Geometry check sheet. Reference: the model listing, model coordinates, mm. A direction names the side the tool comes from. Give positions to 0.01 mm unless a question says otherwise; leave off trailing zeros. Write each loop counter-clockwise with the first axis right and the second up, starting at its lowest first coordinate (ties: lowest second). Pieces come first, ordered by that corner, then holes. Notation, with made-up numbers: (15, -25) -> (35, -25) arc R20 cw to (35, -18) -> close; hole circle Ø8 at (13.25, -33). An arc over 180 degrees is marked (long way). One line per item, written item: value.
from build123d import *

# Parameters (mm, degrees)
SKETCH_2_W          = 38
SKETCH_2_H          = 38
SKETCH_2_R          = 1.15
EXTRUDE_1_DEPTH     = 3.15
EXTRUDE_START       = 3.15
SKETCH_3_W          = 13
SKETCH_3_H          = 13
EXTRUDE_2_DEPTH     = 3.15
EXTRUDE_START_2     = 6.3
SKETCH_4_R          = 6.5
EXTRUDE_3_DEPTH     = 14
CUT_EXTRUDE_START   = 9
SKETCH_5_R          = 32.561017026
SKETCH_5_R_2        = 6
CUT_EXTRUDE_1_DEPTH = 5
SKETCH_6_W          = 10
SKETCH_6_H          = 4.7
EXTRUDE_4_DEPTH     = 6.2
CHAMFER_1_SIZE      = 0.5


with BuildPart() as part:
    # 草图2 → 凸台-拉伸1 (new body)
    with BuildSketch(Plane(origin=(0, 0, 0), x_dir=(1, 0, 0), z_dir=(0, 1, 0))):
        Rectangle(SKETCH_2_W, SKETCH_2_H)
        with Locations((14.25, 14.25)):
            Circle(SKETCH_2_R, mode=Mode.SUBTRACT)
        with Locations((-14.25, 14.25)):
            Circle(SKETCH_2_R, mode=Mode.SUBTRACT)
        with Locations((14.25, -14.25)):
            Circle(SKETCH_2_R, mode=Mode.SUBTRACT)
        with Locations((-14.25, -14.25)):
            Circle(SKETCH_2_R, mode=Mode.SUBTRACT)
    extrude(amount=EXTRUDE_1_DEPTH)

    # 草图3 → 凸台-拉伸2 (add)
    with BuildSketch(Plane(origin=(0, 0, 0), x_dir=(1, 0, 0), z_dir=(0, 1, 0)).offset(EXTRUDE_START)):
        with BuildLine():
            Line((-6.5, -2), (-6.5, 2))
            Line((-6.5, 2), (-9, 2))
            ThreePointArc((-9, 2), (-11, 0), (-9, -2))
            Line((-9, -2), (-6.5, -2))
        make_face()
        Rectangle(SKETCH_3_W, SKETCH_3_H)
        with BuildLine():
            ThreePointArc((9, -2), (11, 0), (9, 2))
            Line((9, 2), (6.5, 2))
            Line((6.5, 2), (6.5, -2))
            Line((6.5, -2), (9, -2))
        make_face()
    extrude(amount=EXTRUDE_2_DEPTH)

    # 草图4 → 凸台-拉伸3 (add)
    with BuildSketch(Plane(origin=(0, 0, 0), x_dir=(1, 0, 0), z_dir=(0, 1, 0)).offset(EXTRUDE_START_2)):
        Circle(SKETCH_4_R)
    extrude(amount=EXTRUDE_3_DEPTH)

    # 草图5 → 切除-拉伸1 (cut)
    with BuildSketch(Plane(origin=(0, 0, 0), x_dir=(1, 0, 0), z_dir=(0, 1, 0)).offset(CUT_EXTRUDE_START)):
        Circle(SKETCH_5_R)
        Circle(SKETCH_5_R_2, mode=Mode.SUBTRACT)
    extrude(amount=CUT_EXTRUDE_1_DEPTH, mode=Mode.SUBTRACT)

    # 草图6 → 凸台-拉伸4 (add)
    with BuildSketch(Plane(origin=(0, 0, 0), x_dir=(1, 0, 0), z_dir=(0, 1, 0))):
        with Locations((0, -12.35)):
            Rectangle(SKETCH_6_W, SKETCH_6_H)
    extrude(amount=-EXTRUDE_4_DEPTH)

    # 倒角1
    chamfer_1_edges = [part.edges().sort_by_distance(p)[0] for p in [
        (-6.5, 20.3, 0),
    ]]
    chamfer(chamfer_1_edges, length=CHAMFER_1_SIZE)


solid = part.part
1) Depth check by flat-ended pin: pin 1 Ø0.9 at (y, z) = (5, -4.5) entering from -X; pin 2 Ø3 at (x, y) = (-7.5, 5.5) entering from -Z; pin 3 Ø5 at (x, y) = (2, -4.5) entering from +Z. Enter the tip coordinate at first touch or a pass-through.
Verdict:
pin 1: x = -6.5
pin 2: z = -6.5
pin 3: z = 14.7
2) Sectioned sample at B-B on x = 14.25. Record the cut outline in (y, z).
Verdict:
outline: (0, -19) -> (3.15, -19) -> (3.15, -15.4) -> (0, -15.4) -> close; (0, -13.1) -> (3.15, -13.1) -> (3.15, 13.1) -> (0, 13.1) -> close; (0, 15.4) -> (3.15, 15.4) -> (3.15, 19) -> (0, 19) -> close
3) Sectioned sample at D-D on y = 11.5. Record the cut outline in (x, z), plus the area to 3 significant figures.
Verdict:
outline: circle Ø12 at (0, 0)
area: 113 mm^2
4) Mould release check, pull along Z, two halves, no side actions. Record for faces 6 (the flat face through (2, 9, 6)), 7 (the flat face through (-8, 5, 2)), 8 (the cylindrical face through (-15.4, 1.6, -14.3)): released by +Z, released by -Z, zero draft, split by the parting line, or undercut.
Verdict:
face 6: zero draft
face 7: released by +Z
face 8: undercut
5) Sectioned sample at C-C on z = 0. Record the cut outline in (x, y).
Verdict:
outline: (-19, 0) -> (19, 0) -> (19, 3.15) -> (11, 3.15) -> (11, 6.3) -> (6.5, 6.3) -> (6.5, 9) -> (6, 9) -> (6, 14) -> (6.5, 14) -> (6.5, 19.8) -> (6, 20.3) -> (-6, 20.3) -> (-6.5, 19.8) -> (-6.5, 14) -> (-6, 14) -> (-6, 9) -> (-6.5, 9) -> (-6.5, 6.3) -> (-11, 6.3) -> (-11, 3.15) -> (-19, 3.15) -> close
6) Sectioned sample at A-A on z = -14.25. Record the cut outline in (x, y), plus the area to 3 significant figures.
Verdict:
outline: (-19, 0) -> (-15.4, 0) -> (-15.4, 3.15) -> (-19, 3.15) -> close; (-13.1, 0) -> (13.1, 0) -> (13.1, 3.15) -> (-13.1, 3.15) -> close; (15.4, 0) -> (19, 0) -> (19, 3.15) -> (15.4, 3.15) -> close
area: 105 mm^2
7) Tool access check on faces 1 (the flat face through (-7, 6.3, -1)), 2 (the cylindrical face through (-5.158, 16.859, 3.955)), 3 (the flat face through (-5, -3, 12)), 4 (the flat face through (8, 5, -2)), 5 (the cylindrical face through (-6, 11, 0)). Record the directions out of +Z, -Z, +X, -X, +Y, -Y that give a thin tool (end or side, any length) a straight path to the whole face; none if there is none.
Verdict:
face 1: -X, +Y
face 2: +Y
face 3: +Z, -Z, -X, -Y
face 4: -Z, +X, +Y
face 5: none
8) Scan lines: probe 1 along X at (y, z) = (2.05, -14.25); probe 2 along Y at (x, z) = (-12, 7). Record each from-to range of solid material in increasing order.
Verdict:
probe 1: -19 to -15.4, -13.1 to 13.1, 15.4 to 19
probe 2: 0 to 3.15
